from build123d import *

# Parameters (mm, degrees)
SKETCH1_W                 = 19.05
SKETCH1_H                 = 57.15
BOSS_EXTRUDE1_DEPTH       = 6.35
M10_CLEARANCE_HOLE1_D     = 11
M10_CLEARANCE_HOLE1_DEPTH = 25.4
M10_CLEARANCE_HOLE1_TIP   = 3.304733405
M8_CLEARANCE_HOLE2_D      = 9
M8_CLEARANCE_HOLE2_DEPTH  = 25.4
M8_CLEARANCE_HOLE2_TIP    = 2.703872786


with BuildPart() as part:
    # Sketch1 → Boss-Extrude1 (new body)
    with BuildSketch(Plane.XY):
        with Locations((0, 61.356)):
            Rectangle(SKETCH1_W, SKETCH1_H)
    extrude(amount=BOSS_EXTRUDE1_DEPTH)

    # M10 Clearance Hole1
    with Locations(Plane.XY.offset(6.35)):
        with Locations((0, 42.306)):
            Hole(M10_CLEARANCE_HOLE1_D / 2, depth=M10_CLEARANCE_HOLE1_DEPTH)
            with Locations((0, 0, -(M10_CLEARANCE_HOLE1_DEPTH + M10_CLEARANCE_HOLE1_TIP / 2))):  # 118° drill point
                Cone(0, M10_CLEARANCE_HOLE1_D / 2, M10_CLEARANCE_HOLE1_TIP, mode=Mode.SUBTRACT)

    # M8 Clearance Hole2
    with Locations(Plane.XY.offset(6.35)):
        with Locations((0, 80.406)):
            Hole(M8_CLEARANCE_HOLE2_D / 2, depth=M8_CLEARANCE_HOLE2_DEPTH)
            with Locations((0, 0, -(M8_CLEARANCE_HOLE2_DEPTH + M8_CLEARANCE_HOLE2_TIP / 2))):  # 118° drill point
                Cone(0, M8_CLEARANCE_HOLE2_D / 2, M8_CLEARANCE_HOLE2_TIP, mode=Mode.SUBTRACT)


solid = part.part
Here's how the part is built. I have some questions about the finished solid (model axes, mm). Round coordinates to 2 decimals unless told otherwise and drop trailing zeros. Loops run counter-clockwise (first coordinate to the right, second up) from the corner with the lowest first, then second, coordinate; pieces in that order, holes last. Notation, with made-up numbers: (-34, 74.5) -> (-5, 74.5) arc R20 cw to (-5, 92.5) -> close; hole circle Ø11 at (48, 58). An arc over 180 degrees is marked (long way). Write each question's results on one line, items separated by ' | '.
(1) If we section it at C-C, the plane z = 4.25: List the corners of the cut face in (x, y) for me (3 decimals).
Worked answers:
outline: (-9.525, 32.781) -> (9.525, 32.781) -> (9.525, 89.931) -> (-9.525, 89.931) -> close; hole circle Ø11 at (0, 42.306); hole circle Ø9 at (0, 80.406)
(2) We'd pull the mould along Y, two halves only. Please class faces 1 (the face through (0, 89.931, 3)), 2 (the face through (0.586, 84.868, 3.131)), 3 (the face through (0, 62, 0)): released by +Y, released by -Y, zero draft, split by the parting line, or undercut.
Worked answers:
face 1: released by +Y | face 2: undercut | face 3: zero draft
(3) If we section it at D-D, the plane x = 3: List the corners of the cut face in (y, z) for me.
Worked answers:
outline: (32.78, 0) -> (37.7, 0) -> (37.7, 6.35) -> (32.78, 6.35) -> close; (46.92, 0) -> (77.05, 0) -> (77.05, 6.35) -> (46.92, 6.35) -> close; (83.76, 0) -> (89.93, 0) -> (89.93, 6.35) -> (83.76, 6.35) -> close
(4) For P1, Ø9, axis at x = 0, y = 42.306, coming from the -Z side, with a flat end and sliding along its axis, tell me the tip position at first contact or that it passes through.
Worked answers:
P1: through
(5) If we section it at A-A, the plane x = 0: List the corners of the cut face in (y, z) for me.
Worked answers:
outline: (32.78, 0) -> (36.81, 0) -> (36.81, 6.35) -> (32.78, 6.35) -> close; (47.81, 0) -> (75.91, 0) -> (75.91, 6.35) -> (47.81, 6.35) -> close; (84.91, 0) -> (89.93, 0) -> (89.93, 6.35) -> (84.91, 6.35) -> close
(6) If I drill on L1, parallel to Y at x = 0, z = 4; L2, parallel to Y at x = 1.5, z = 4; L3, parallel to X at y = 44, z = 4.75 (3 decimals), over which ranges is the centre line in solid material (lowest first)?
Worked answers:
L1: 32.78 to 36.81, 47.81 to 75.91, 84.91 to 89.93 | L2: 32.78 to 37.01, 47.6 to 76.16, 84.65 to 89.93 | L3: -9.525 to -5.233, 5.233 to 9.525
(7) If we section it at B-B, the plane y = 83.5: List the corners of the cut face in (x, z) for me (3 decimals).
Worked answers:
outline: (-9.525, 0) -> (-3.268, 0) -> (-3.268, 6.35) -> (-9.525, 6.35) -> close; (3.268, 0) -> (9.525, 0) -> (9.525, 6.35) -> (3.268, 6.35) -> close
